Check sheet for the modelled part. Datum: model origin and axes. Units: mm. Give positions to 0.01 mm unless a question says otherwise; leave off trailing zeros. Order: outer loops, then holes, each group sorted by start corner. A loop starts at its lowest first (then second) coordinate and runs counter-clockwise, first axis right, second up.
Item 1: Sectioned sample at A-A on x = 44.5. Record the boundary of the cut face in (y, z).
Item 2: Material ranges on line 1 along Y through (x, z) = (-97, 1.5); line 2 along Y through (x, z) = (-73, 0.7), recorded low to high.
Item 3: Gauge pin test, flat end, axial feed: P1, Ø3.5, axis at x = -91, y = 11.8, coming from the +Z side. Record the tip position at first contact, or that the pin passes through.
Item 4: Sectioned sample at B-B on z = 0.35. Count the separate pieces of the cut face and the enclosed holes in it, and give its area (3 significant figures).
from build123d import *

# Parameters (mm, degrees)
SKETCH_1_W          = 200
SKETCH_1_H          = 39.4
SKETCH_1_R          = 1.55
SKETCH_1_W_2        = 2
SKETCH_1_H_2        = 18
EXTRUDE_1_DEPTH     = 2
CUT_EXTRUDE_1_DEPTH = 3


with BuildPart() as part:
    # 草图1 → 凸台-拉伸1 (new body)
    with BuildSketch(Plane.XY):
        Rectangle(SKETCH_1_W, SKETCH_1_H)
        with Locations((97, 1.43)):
            Circle(SKETCH_1_R, mode=Mode.SUBTRACT)
        with Locations((97, -8.57)):
            Circle(SKETCH_1_R, mode=Mode.SUBTRACT)
        with Locations((58, 2)):
            Circle(SKETCH_1_R, mode=Mode.SUBTRACT)
        with Locations((58, -8)):
            Circle(SKETCH_1_R, mode=Mode.SUBTRACT)
        with Locations((-97, 1.43)):
            Circle(SKETCH_1_R, mode=Mode.SUBTRACT)
        with Locations((-97, -8.57)):
            Circle(SKETCH_1_R, mode=Mode.SUBTRACT)
        with Locations((-58, -8)):
            Circle(SKETCH_1_R, mode=Mode.SUBTRACT)
        with Locations((-58, 2)):
            Circle(SKETCH_1_R, mode=Mode.SUBTRACT)
        with Locations((73, 11.8)):
            Circle(SKETCH_1_R, mode=Mode.SUBTRACT)
        with Locations((73, 1.8)):
            Circle(SKETCH_1_R, mode=Mode.SUBTRACT)
        with Locations((-73, 11.8)):
            Circle(SKETCH_1_R, mode=Mode.SUBTRACT)
        with Locations((-73, 1.8)):
            Circle(SKETCH_1_R, mode=Mode.SUBTRACT)
        with Locations((91, 11.8)):
            Circle(SKETCH_1_R, mode=Mode.SUBTRACT)
        with Locations((91, 1.8)):
            Circle(SKETCH_1_R, mode=Mode.SUBTRACT)
        with Locations((-91, 1.8)):
            Circle(SKETCH_1_R, mode=Mode.SUBTRACT)
        with Locations((-91, 11.8)):
            Circle(SKETCH_1_R, mode=Mode.SUBTRACT)
        with Locations((87, 1.8)):
            Rectangle(SKETCH_1_W_2, SKETCH_1_H_2, mode=Mode.SUBTRACT)
        with Locations((-87, 1.8)):
            Rectangle(SKETCH_1_W_2, SKETCH_1_H_2, mode=Mode.SUBTRACT)
        with Locations((77, 1.8)):
            Rectangle(SKETCH_1_W_2, SKETCH_1_H_2, mode=Mode.SUBTRACT)
        with Locations((-77, 1.8)):
            Rectangle(SKETCH_1_W_2, SKETCH_1_H_2, mode=Mode.SUBTRACT)
    extrude(amount=EXTRUDE_1_DEPTH)

    # 草图2 → 切除-拉伸1 (cut, through all)
    with BuildSketch(Plane.XY.offset(2)):
        with BuildLine():
            Line((-50.932586808, 14.42388858), (-37.550945645, -11.894165105))
            ThreePointArc((-37.550945645, -11.894165105), (-38.772782628, -15.643779248), (-42.522396771, -14.421942266))
            Line((-42.522396771, -14.421942266), (-55.904037934, 11.89611142))
            ThreePointArc((-55.904037934, 11.89611142), (-54.682200951, 15.645725563), (-50.932586808, 14.42388858))
        make_face()
        with BuildLine():
            Line((-40.932586808, 14.42388858), (-27.550945645, -11.894165105))
            ThreePointArc((-27.550945645, -11.894165105), (-28.772782628, -15.643779248), (-32.522396771, -14.421942266))
            Line((-32.522396771, -14.421942266), (-45.904037934, 11.89611142))
            ThreePointArc((-45.904037934, 11.89611142), (-44.682200951, 15.645725563), (-40.932586808, 14.42388858))
        make_face()
        with BuildLine():
            Line((-30.932586808, 14.42388858), (-17.550945645, -11.894165105))
            ThreePointArc((-17.550945645, -11.894165105), (-18.772782628, -15.643779248), (-22.522396771, -14.421942266))
            Line((-22.522396771, -14.421942266), (-35.904037934, 11.89611142))
            ThreePointArc((-35.904037934, 11.89611142), (-34.682200951, 15.645725563), (-30.932586808, 14.42388858))
        make_face()
        with BuildLine():
            Line((-20.932586808, 14.42388858), (-7.550945645, -11.894165105))
            ThreePointArc((-7.550945645, -11.894165105), (-8.772782628, -15.643779248), (-12.522396771, -14.421942266))
            Line((-12.522396771, -14.421942266), (-25.904037934, 11.89611142))
            ThreePointArc((-25.904037934, 11.89611142), (-24.682200951, 15.645725563), (-20.932586808, 14.42388858))
        make_face()
        with BuildLine():
            Line((-10.932586808, 14.42388858), (2.449054355, -11.894165105))
            ThreePointArc((2.449054355, -11.894165105), (1.227217372, -15.643779248), (-2.522396771, -14.421942266))
            Line((-2.522396771, -14.421942266), (-15.904037934, 11.89611142))
            ThreePointArc((-15.904037934, 11.89611142), (-14.682200951, 15.645725563), (-10.932586808, 14.42388858))
        make_face()
        with BuildLine():
            Line((-0.932586808, 14.42388858), (12.449054355, -11.894165105))
            ThreePointArc((12.449054355, -11.894165105), (11.227217372, -15.643779248), (7.477603229, -14.421942266))
            Line((7.477603229, -14.421942266), (-5.904037934, 11.89611142))
            ThreePointArc((-5.904037934, 11.89611142), (-4.682200951, 15.645725563), (-0.932586808, 14.42388858))
        make_face()
        with BuildLine():
            Line((9.067413192, 14.42388858), (22.449054355, -11.894165105))
            ThreePointArc((22.449054355, -11.894165105), (21.227217372, -15.643779248), (17.477603229, -14.421942266))
            Line((17.477603229, -14.421942266), (4.095962066, 11.89611142))
            ThreePointArc((4.095962066, 11.89611142), (5.317799049, 15.645725563), (9.067413192, 14.42388858))
        make_face()
        with BuildLine():
            Line((19.067413192, 14.42388858), (32.449054355, -11.894165105))
            ThreePointArc((32.449054355, -11.894165105), (31.227217372, -15.643779248), (27.477603229, -14.421942266))
            Line((27.477603229, -14.421942266), (14.095962066, 11.89611142))
            ThreePointArc((14.095962066, 11.89611142), (15.317799049, 15.645725563), (19.067413192, 14.42388858))
        make_face()
        with BuildLine():
            Line((29.067413192, 14.42388858), (42.449054355, -11.894165105))
            ThreePointArc((42.449054355, -11.894165105), (41.227217372, -15.643779248), (37.477603229, -14.421942266))
            Line((37.477603229, -14.421942266), (24.095962066, 11.89611142))
            ThreePointArc((24.095962066, 11.89611142), (25.317799049, 15.645725563), (29.067413192, 14.42388858))
        make_face()
        with BuildLine():
            Line((39.067413192, 14.42388858), (52.449054355, -11.894165105))
            ThreePointArc((52.449054355, -11.894165105), (51.227217372, -15.643779248), (47.477603229, -14.421942266))
            Line((47.477603229, -14.421942266), (34.095962066, 11.89611142))
            ThreePointArc((34.095962066, 11.89611142), (35.317799049, 15.645725563), (39.067413192, 14.42388858))
        make_face()
    extrude(amount=-CUT_EXTRUDE_1_DEPTH, mode=Mode.SUBTRACT)


solid = part.part
Report:
1. outline: (-19.7, 0) - (-8.57, 0) - (-8.57, 2) - (-19.7, 2) - close; (3.74, 0) - (19.7, 0) - (19.7, 2) - (3.74, 2) - close
2. line 1: y = -19.7 to -10.12, -7.02 to -0.12, 2.98 to 19.7
2. line 2: y = -19.7 to 0.25, 3.35 to 10.25, 13.35 to 19.7
3. P1: stops at z = 2
4. separate pieces: 1
4. enclosed holes: 30
4. area: 5,720 mm2
